from build123d import *

# Parameters (mm, degrees)
PCB_R              = 1.75
BOARD_DEPTH        = 1.6
GIGE_W             = 21.29
GIGE_H             = 17.01
ETHERNETPORT_DEPTH = 14
HDMI_W             = 10.5
HDMI_H             = 14.5
HDMIPORT_DEPTH     = 6.7
SKETCH9_W          = 19
SKETCH9_H          = 19
FPGAANDFAN_DEPTH   = 14.4


with BuildPart() as part:
    # pcb → board (new body)
    with BuildSketch(Plane.XY.offset(-31.428393775)):
        with BuildLine():
            Line((91.850829578, -91.451333311), (91.850829578, -136.451333311))
            ThreePointArc((91.850829578, -136.451333311), (90.532810093, -139.633313826), (87.350829578, -140.951333311))
            Line((87.350829578, -140.951333311), (0.210829578, -140.951333311))
            ThreePointArc((0.210829578, -140.951333311), (-2.971150937, -139.633313826), (-4.289170422, -136.451333311))
            Line((-4.289170422, -136.451333311), (-4.289170422, -91.451333311))
            ThreePointArc((-4.289170422, -91.451333311), (-2.923602921, -88.384143861), (0.210829578, -87.180915442))
            Line((0.210829578, -87.180915442), (87.350829578, -86.951333311))
            ThreePointArc((87.350829578, -86.951333311), (90.532810093, -88.269352795), (91.850829578, -91.451333311))
        make_face()
        with Locations((87.350829578, -136.451333311)):
            Circle(PCB_R, mode=Mode.SUBTRACT)
        with Locations((87.350829578, -91.451333311)):
            Circle(PCB_R, mode=Mode.SUBTRACT)
        with Locations((0.210829578, -91.451333311)):
            Circle(PCB_R, mode=Mode.SUBTRACT)
        with Locations((0.210829578, -136.451333311)):
            Circle(PCB_R, mode=Mode.SUBTRACT)
    extrude(amount=BOARD_DEPTH)

    # gige → ethernetport (add)
    with BuildSketch(Plane.XY.offset(-29.828393775)):
        with Locations((81.505829578, -104.516333311)):
            Rectangle(GIGE_W, GIGE_H)
    extrude(amount=ETHERNETPORT_DEPTH)

    # hdmi → hdmiport (add)
    with BuildSketch(Plane.XY.offset(-29.828393775)):
        with Locations((86.600829578, -124.441333311)):
            Rectangle(HDMI_W, HDMI_H)
    extrude(amount=HDMIPORT_DEPTH)

    # Sketch9 → FPGAandFan (add)
    with BuildSketch(Plane.XY.offset(-29.828393775)):
        with Locations((50.620829578, -114.802468161)):
            Rectangle(SKETCH9_W, SKETCH9_H)
    extrude(amount=FPGAANDFAN_DEPTH)


solid = part.part
Can you work these out from the model? Positions are in its coordinate system, mm. A direction names the side the tool comes from. Give positions to 0.01 mm unless a question says otherwise; leave off trailing zeros. Order: outer loops, then holes, each group sorted by start corner. A loop starts at its lowest first (then second) coordinate and runs counter-clockwise, first axis right, second up. Notation, with made-up numbers: M 87.5,54.5 L 123.5,54.5 A33 ccw 123.5,89.5 Z; hole C 38.5,19.25 d7. An arc over 180 degrees is marked long. Use a Markdown table: item, result. Add a question column.
Item 1: Suppose I cut it at D-D (y = -128). List the corners of the cut face in (x, z) for me, then the cut area to 3 significant figures.
Item 2: If I drill on L1, parallel to Y at x = 84, z = -26.75; L2, parallel to Z at x = 50, y = -101.5; L3, parallel to Y at x = 74, z = -22, over which ranges is the centre line in solid material (lowest first)? Write a range as [from, to].
Item 3: Will these pins go through, and if not, where does the flat tip stop? pin 1 (5 mm diameter, centred on x = 81, y = -104, fed in from +Z); pin 2 (4 mm diameter, centred on x = 8.5, y = -107.5, fed in from +Z); pin 3 (1 mm diameter, centred on y = -116, z = -29.5, fed in from +X).
Item 4: Suppose I cut it at B-B (y = -114). List the corners of the cut face in (x, z) for me, then the cut area to 3 significant figures.
Item 5: Suppose I cut it at A-A (z = -24.25). List the corners of the cut face in (x, y) for me.
Item 6: For faces 1 (the flat face through (87, -124, -23.128)), 2 (the flat face through (87, -131.691, -27)), 3 (the flat face through (41.121, -115, -23)), 4 (the flat face through (81, -96.011, -23)), 5 (the flat face through (81, -104, -15.828)), which set-ups out of +Z, -Z, +X, -X, +Y, -Y let a thin tool reach every point of the face, with its end or its side?
Item 7: Suppose I cut it at C-C (x = 50.5). List the corners of the cut face in (y, z) for me, then the cut area to 3 significant figures.
Answer sheet:
| question | item | result |
|---|---|---|
| 1 | outline | M -4.29,-31.43 L 91.85,-31.43 L 91.85,-23.13 L 81.35,-23.13 L 81.35,-29.83 L -4.29,-29.83 Z |
| 1 | area | 224 mm² |
| 2 | L1 | y = [-131.69, -117.19], [-113.02, -96.01] |
| 2 | L2 | z = [-31.43, -29.83] |
| 2 | L3 | y = [-113.02, -96.01] |
| 3 | pin 1 | stops at z = -15.83 |
| 3 | pin 2 | stops at z = -29.83 |
| 3 | pin 3 | stops at x = 91.85 |
| 4 | outline | M -4.29,-31.43 L 91.85,-31.43 L 91.85,-29.83 L 60.12,-29.83 L 60.12,-15.43 L 41.12,-15.43 L 41.12,-29.83 L -4.29,-29.83 Z |
| 4 | area | 427 mm² |
| 5 | outline | M 41.12,-124.3 L 60.12,-124.3 L 60.12,-105.3 L 41.12,-105.3 Z; M 70.86,-113.02 L 92.15,-113.02 L 92.15,-96.01 L 70.86,-96.01 Z; M 81.35,-131.69 L 91.85,-131.69 L 91.85,-117.19 L 81.35,-117.19 Z |
| 6 | face 1 | +Z, +X, -Y |
| 6 | face 2 | +Z, +X, -X, -Y |
| 6 | face 3 | +Z, -X, +Y, -Y |
| 6 | face 4 | +Z, +X, -X, +Y |
| 6 | face 5 | +Z, +X, +Y, -Y |
| 7 | outline | M -140.95,-31.43 L -87.05,-31.43 L -87.05,-29.83 L -105.3,-29.83 L -105.3,-15.43 L -124.3,-15.43 L -124.3,-29.83 L -140.95,-29.83 Z |
| 7 | area | 360 mm² |
